The drawing under review shows one solid part. Ordinate dimensions are in mm from its lowest x, y, z. A direction names the side the tool comes from. Coordinates: 2 decimals unless noted, no trailing zeros. Write each loop counter-clockwise with the first axis right and the second up, starting at its lowest first coordinate (ties: lowest second). Pieces come first, ordered by that corner, then holes.
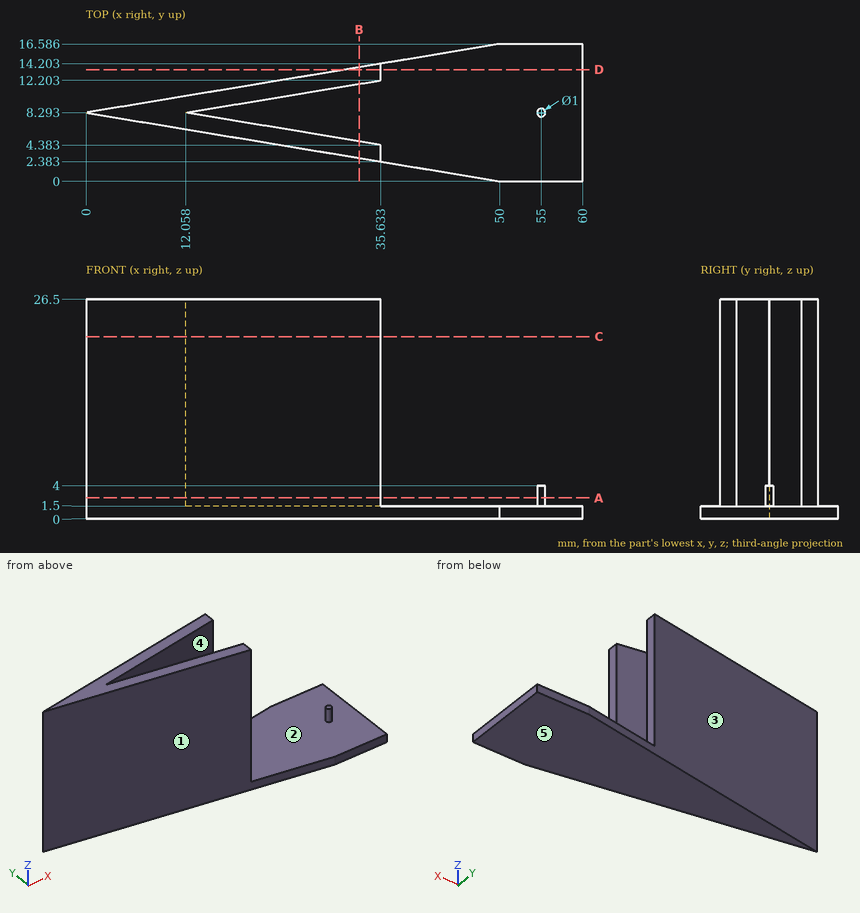
1) Consider section B-B (x = 33). Give the boundary of the cut face in (y, z), then the cut area to 3 significant figures.
2) Consider section D-D (y = 13.5). Give the boundary of the cut face in (x, z), then the cut area to 3 significant figures.
3) For L1, parallel to Z at x = 43, y = 3.75; L2, parallel to Z at x = 55, y = 8.25; L3, parallel to Y at x = 33, z = 9.5, list the stretches that pass through material, from the lowest coordinate up.
4) Consider section A-A (z = 2.5). Give the boundary of the cut face in (x, y), then the cut area to 3 significant figures.
5) Tool access review of the marked faces 1 and 2: name each direction out of +Z, -Z, +X, -X, +Y, -Y from which nothing blocks a thin tool from reaching the whole face with its end or side.
6) Clearance check with flat-ended pins moving along their axes: P1, Ø1.5, axis at x = 25, z = 15.5, coming from the +Y side; P2, Ø2, axis at y = 3.5, z = 20, coming from the +X side; P3, Ø5, axis at x = 19.5, z = 9, coming from the -Y side. State where each tip first meets the part, or that it passes through.
7) The part is to be moulded in two halves that separate along Y. For the marked faces 3, 4 and 5, say which applies: pulls with the +Y half, pulls with the -Y half, needs draft (parallel to the pull), parting line crosses it, or undercut.
8) Consider section C-C (z = 22). Give the boundary of the cut face in (x, y), then the cut area to 3 significant figures.
Results:
1. outline: (2.82, 0) - (13.77, 0) - (13.77, 26.5) - (11.77, 26.5) - (11.77, 1.5) - (4.82, 1.5) - (4.82, 26.5) - (2.82, 26.5) - close
1. area: 116 mm2
2. outline: (31.39, 0) - (60, 0) - (60, 1.5) - (35.63, 1.5) - (35.63, 26.5) - (31.39, 26.5) - close
2. area: 149 mm2
3. L1: z = 0 to 1.5
3. L2: z = 0 to 4
3. L3: y = 2.82 to 4.82, 11.77 to 13.77
4. outline: (0, 8.29) - (35.63, 2.38) - (35.63, 4.38) - (12.06, 8.29) - (35.63, 12.2) - (35.63, 14.2) - close; circle Ø1 at (55, 8.29)
4. area: 119 mm2
5. face 1: +Z, -Z, -X, -Y
5. face 2: +Z
6. P1: stops at y = 12.56
6. P2: stops at x = 35.63
6. P3: stops at y = 4.64
7. face 3: pulls with the +Y half
7. face 4: undercut
7. face 5: needs draft
8. outline: (0, 8.29) - (35.63, 2.38) - (35.63, 4.38) - (12.06, 8.29) - (35.63, 12.2) - (35.63, 14.2) - close
8. area: 118 mm2
